Here's the drawing with two shaded views (mm, measured from the low corner). I have some questions. A direction names the side the tool comes from. Round coordinates to 2 decimals unless told otherwise and drop trailing zeros. Order: outer loops, then holes, each group sorted by start corner. A loop starts at its lowest first (then second) coordinate and runs counter-clockwise, first axis right, second up. Notation, with made-up numbers: (9, -37.5) - (41, -37.5) arc R10 cw to (41, -20.5) - close; hole circle Ø6 at (26, 16). An arc over 180 degrees is marked (long way). One line per item, written item: value.
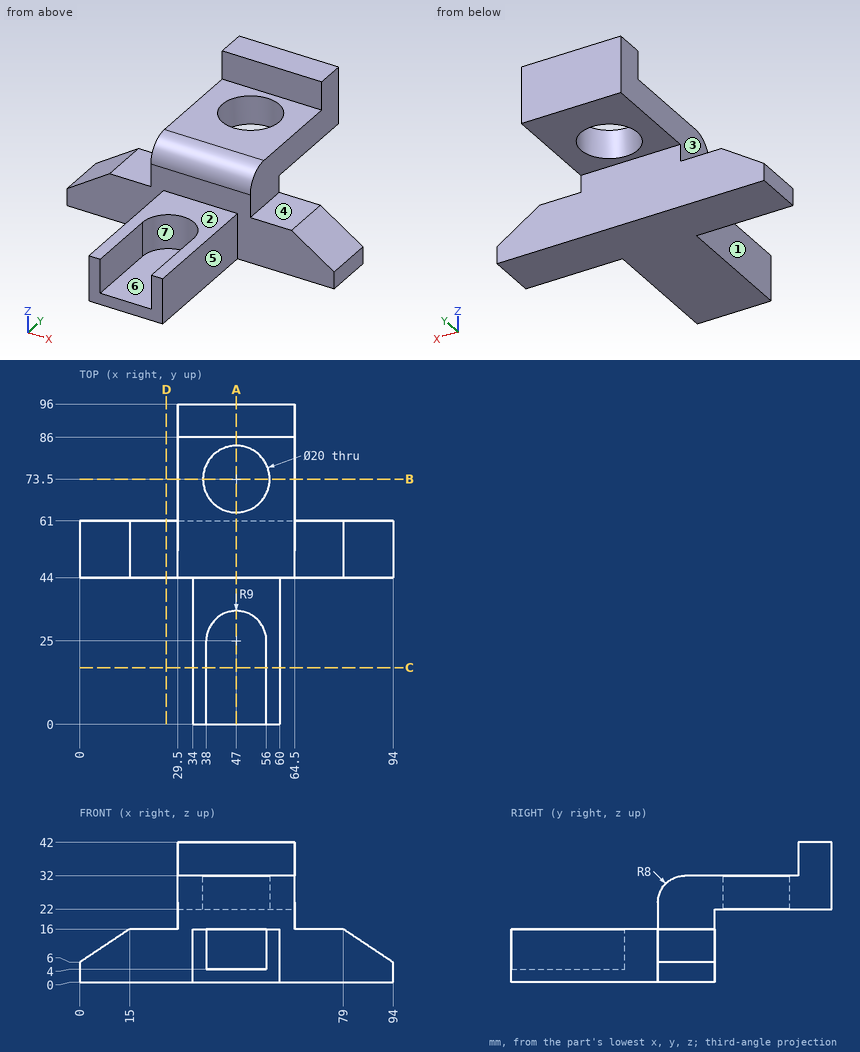
Q1. If we section it at C-C, the plane y = 17: Please give me the cut outline in (x, z).
Results list:
outline: (34, 0) - (60, 0) - (60, 16) - (56, 16) - (56, 4) - (38, 4) - (38, 16) - (34, 16) - close
Q2. Will these pins go through, and if not, where does the flat tip stop? pin 1 (1.5 mm diameter, centred on y = 60, z = 10.5, fed in from +X) (3 decimals); pin 2 (13 mm diameter, centred on y = 12, z = 8, fed in from -X); pin 3 (9.5 mm diameter, centred on y = 12, z = 11, fed in from +X).
Results list:
pin 1: x = 88.375
pin 2: x = 34
pin 3: x = 60
Q3. Which directions (+Z, -Z, +X, -X, +Y, -Y) give clear straight access to the entire face, cutting with the end or side of a thin tool? Please do the marked faces 1, 2 and 3.
Results list:
face 1: +Z, -Z, -X, -Y
face 2: +Z, +X, -X, -Y
face 3: +Z, -X, +Y, -Y
Q4. If I drill on line 1 along Y through (x, z) = (47, 24.5); line 2 along Z through (x, y) = (37.5, 41); line 3 along Z through (x, y) = (42, 86.5), over which ranges is the centre line in solid material (lowest first)?
Results list:
line 1: 44.02 to 63.5, 83.5 to 96
line 2: 0 to 16
line 3: 22 to 42
Q5. If we section it at A-A, the plane x = 47: Please give me the cut outline in (y, z), then the cut area to 3 significant figures.
Results list:
outline: (0, 0) - (61, 0) - (61, 22) - (63.5, 22) - (63.5, 32) - (52, 32) arc R8 ccw to (44, 24) - (44, 16) - (34, 16) - (34, 4) - (0, 4) - close; (83.5, 22) - (96, 22) - (96, 42) - (86, 42) - (86, 32) - (83.5, 32) - close
area: 1,080 mm²
Q6. If we section it at B-B, the plane y = 73.5: Please give me the cut outline in (x, z).
Results list:
outline: (29.5, 22) - (37, 22) - (37, 32) - (29.5, 32) - close; (57, 22) - (64.5, 22) - (64.5, 32) - (57, 32) - close
Q7. If we section it at D-D, the plane x = 26: Please give me the cut outline in (y, z).
Results list:
outline: (44, 0) - (61, 0) - (61, 16) - (44, 16) - close
Q8. We'd pull the mould along X, two halves only. Please class the marked faces 4, 5, 6 and 7: released by +X, released by -X, zero draft, split by the parting line, or undercut.
Results list:
face 4: zero draft
face 5: released by +X
face 6: undercut
face 7: undercut
